```python
from build123d import *

# Parameters (mm, degrees)
BOSS_EXTRUDE1_DEPTH = 8.571428571
SCALE1_SCALE        = 0.35
SKETCH4_R           = 5
SKETCH4_R_2         = 2.5
CUT_EXTRUDE1_DEPTH  = 3


with BuildPart() as part:
    # Sketch1 → Boss-Extrude1 (new body)
    with BuildSketch(Plane.XY):
        with BuildLine():
            Line((58.123111297, 76.596610431), (85.302723175, 163.49128587))
            ThreePointArc((85.302723175, 163.49128587), (104.096629497, 173.329430267), (113.934773893, 154.535523945))
            Line((113.934773893, 154.535523945), (86.755162015, 67.640848506))
            ThreePointArc((86.755162015, 67.640848506), (72.021658749, 37.591328154), (48.934001898, 13.363041111))
            Line((48.934001898, 13.363041111), (5.217217629, -20.341042592))
            ThreePointArc((5.217217629, -20.341042592), (2.676812565, -23.236266616), (1.419146317, -26.876906073))
            ThreePointArc((1.419146317, -26.876906073), (-8.076031964, -43.216564777), (-26.293681135, -48.242509049))
            ThreePointArc((-26.293681135, -48.242509049), (-30.134490911, -48.532613024), (-33.580740804, -50.252886758))
            Line((-33.580740804, -50.252886758), (-58.231756308, -69.257941768))
            ThreePointArc((-58.231756308, -69.257941768), (-73.309006949, -114.009842439), (-37.733455904, -145.065216667))
            Line((-37.733455904, -145.065216667), (-12.872173051, -148.280481329))
            ThreePointArc((-12.872173051, -148.280481329), (0.08003541, -165.080490138), (-16.719973399, -178.032698599))
            Line((-16.719973399, -178.032698599), (-41.581256252, -174.817433937))
            ThreePointArc((-41.581256252, -174.817433937), (-102.268960976, -121.840619078), (-76.548945176, -45.499141462))
            Line((-76.548945176, -45.499141462), (-51.897929672, -26.494086452))
            ThreePointArc((-51.897929672, -26.494086452), (-49.357524607, -23.598862428), (-48.09985836, -19.958222971))
            ThreePointArc((-48.09985836, -19.958222971), (-38.604680078, -3.618564267), (-20.387030907, 1.407380005))
            ThreePointArc((-20.387030907, 1.407380005), (-16.546221132, 1.69748398), (-13.099971239, 3.417757714))
            Line((-13.099971239, 3.417757714), (30.61681303, 37.121841417))
            ThreePointArc((30.61681303, 37.121841417), (47.407836194, 54.742413811), (58.123111297, 76.596610431))
        make_face()
    extrude(amount=BOSS_EXTRUDE1_DEPTH)


with BuildPart() as part_1:
    # Scale1: scaled about (-2.128000964, -18.472945164, 4.285714286)
    add(part.part.scale(SCALE1_SCALE).moved(Location((-1.383200627, -12.007414357, 2.785714286))))

    # Sketch4 → Cut-Extrude1 (cut)
    with BuildSketch(Plane.XY.offset(5.785714286)):
        with Locations((-9.552325234, -20.203561939)):
            Circle(SKETCH4_R)
        with Locations((33.48336136, 43.647277361)):
            Circle(SKETCH4_R_2)
    extrude(amount=-CUT_EXTRUDE1_DEPTH, mode=Mode.SUBTRACT)


solid = part_1.part
```
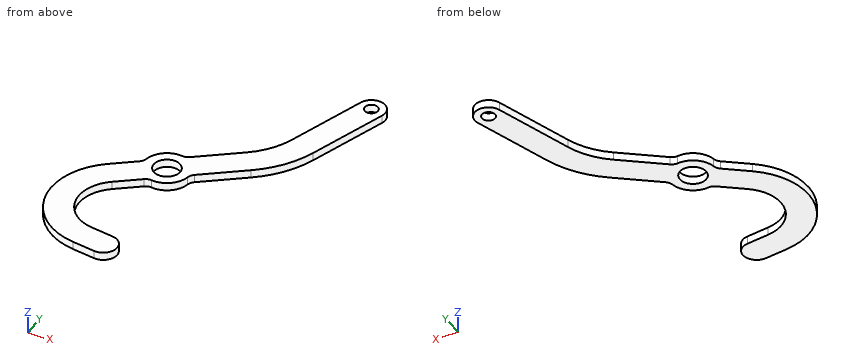
Part model, mm, in its own coordinate system. Round coordinates to 2 decimals unless told otherwise and drop trailing zeros. Write each loop counter-clockwise with the first axis right and the second up, starting at its lowest first coordinate (ties: lowest second). Pieces come first, ordered by that corner, then holes.
Item 1: Cut at A-A, the plane y = -16.5. Give the cut face in (x, z), plus the area to 3 significant figures.
Results:
outline: (-17.48, 2.79) - (-12.91, 2.79) - (-12.91, 5.79) - (-17.48, 5.79) - close; (-6.19, 2.79) - (3.85, 2.79) - (3.85, 5.79) - (-6.19, 5.79) - close
area: 43.8 mm2
Item 2: Cut at B-B, the plane z = 3.75. Count the separate pieces of the cut face and the enclosed holes in it, plus the area to 3 significant figures.
Results:
separate pieces: 1
enclosed holes: 2
area: 1,690 mm2
Item 3: Drop flat-ended pins along their axis: pin 1 Ø4.5 at (x, y) = (33.48, 43.65) entering from +Z; pin 2 Ø1.5 at (x, z) = (-7, 3.5) entering from +Y. Give the stop position or say it passes through.
Results:
pin 1: passes through
pin 2: stops at y = -11.01
Item 4: Cut at C-C, the plane x = 5. Give the cut face in (y, z).
Results:
outline: (-15.61, 2.79) - (-2.36, 2.79) - (-2.36, 5.79) - (-15.61, 5.79) - close
Item 5: Cut at D-D, the plane y = -58.5. Give the cut face in (x, z), plus the area to 3 significant figures.
Results:
outline: (-35.8, 2.79) - (-23.25, 2.79) - (-23.25, 5.79) - (-35.8, 5.79) - close
area: 37.6 mm2
Item 6: Probe L1, parallel to Y at x = -18.5, z = 4.15; L2, parallel to Y at x = -25, z = 4.35; L3, parallel to Y at x = -5, z = 5.4. List the from-to ranges inside material, lowest first.
Results:
L1: y = -72.73 to -61.72, -33.73 to -19.96
L2: y = -70.21 to -56.37, -39.69 to -25.48
L3: y = -74.12 to -64.1, -27.68 to -22.27, -18.14 to -10.06
